from build123d import *

# Parameters (mm, degrees)
EXTRUDE1_DEPTH          = 20.6375
EXTRUDE1_DEPTH_BACK     = 20.6375
SKETCH2_R               = 4.0005
SKETCH2_R_2             = 1.1938
CUT_EXTRUDE1_DEPTH      = 20.6375
CUT_EXTRUDE1_DEPTH_BACK = 20.6375
SKETCH3_R               = 1.1938
CUT_EXTRUDE2_DEPTH      = 23.62886
CUT_EXTRUDE2_DEPTH_BACK = 23.62886
FILLET1_R               = 1.5875


with BuildPart() as part:
    # Sketch1 → Extrude1 (new body, two sides)
    with BuildSketch(Plane(origin=(0, 0, 0), x_dir=(0, 0, -1), z_dir=(1, 0, 0))) as extrude1_sk:
        with BuildLine():
            Line((-20.85086, 0), (20.85086, 0))
            ThreePointArc((20.85086, 0), (22.108095857, 0.520764143), (22.62886, 1.778))
            Line((22.62886, 1.778), (22.62886, 23.8252))
            Line((22.62886, 23.8252), (21.10486, 23.8252))
            Line((21.10486, 23.8252), (21.10486, 1.778))
            ThreePointArc((21.10486, 1.778), (21.030465122, 1.598394878), (20.85086, 1.524))
            Line((20.85086, 1.524), (-20.85086, 1.524))
            ThreePointArc((-20.85086, 1.524), (-21.030465122, 1.598394878), (-21.10486, 1.778))
            Line((-21.10486, 1.778), (-21.10486, 23.8252))
            Line((-21.10486, 23.8252), (-22.62886, 23.8252))
            Line((-22.62886, 23.8252), (-22.62886, 1.778))
            ThreePointArc((-22.62886, 1.778), (-22.108095857, 0.520764143), (-20.85086, 0))
        make_face()
    extrude(amount=EXTRUDE1_DEPTH)
    extrude(extrude1_sk.sketch, amount=-EXTRUDE1_DEPTH_BACK)

    # Sketch2 → Cut-Extrude1 (cut, two sides)
    with BuildSketch(Plane(origin=(0, 0, 0), x_dir=(1, 0, 0), z_dir=(0, 1, 0))) as cut_extrude1_sk:
        with Locations(Location((-8.3312, 0, 0), (0, 0, 270))):  # turned: the seam where the file's is
            Circle(SKETCH2_R)
        with Locations(Location((8.3312, 0, 0), (0, 0, 270))):  # turned: the seam where the file's is
            Circle(SKETCH2_R)
        with Locations(Location((16.6624, 0, 0), (0, 0, 270))):  # turned: the seam where the file's is
            Circle(SKETCH2_R_2)
        with Locations(Location((-16.6624, 0, 0), (0, 0, 270))):  # turned: the seam where the file's is
            Circle(SKETCH2_R_2)
        with Locations(Location((-8.3312, 8.3312, 0), (0, 0, 270))):  # turned: the seam where the file's is
            Circle(SKETCH2_R_2)
        with Locations(Location((8.3312, 8.3312, 0), (0, 0, 270))):  # turned: the seam where the file's is
            Circle(SKETCH2_R_2)
        with Locations(Location((-8.3312, -8.3312, 0), (0, 0, 270))):  # turned: the seam where the file's is
            Circle(SKETCH2_R_2)
        with Locations(Location((8.3312, -8.3312, 0), (0, 0, 270))):  # turned: the seam where the file's is
            Circle(SKETCH2_R_2)
        with Locations(Location((0, 0, 0), (0, 0, 270))):  # turned: the seam where the file's is
            Circle(SKETCH2_R_2)
    extrude(amount=CUT_EXTRUDE1_DEPTH, mode=Mode.SUBTRACT)
    extrude(cut_extrude1_sk.sketch, amount=-CUT_EXTRUDE1_DEPTH_BACK, mode=Mode.SUBTRACT)

    # Sketch3 → Cut-Extrude2 (cut, two sides)
    with BuildSketch(Plane.XY) as cut_extrude2_sk:
        with Locations((-17.8689, 13.8938)):
            Circle(SKETCH3_R)
        with Locations((-9.9187, 13.8938)):
            Circle(SKETCH3_R)
        with Locations((9.9187, 13.8938)):
            Circle(SKETCH3_R)
        with Locations((17.8689, 13.8938)):
            Circle(SKETCH3_R)
    extrude(amount=CUT_EXTRUDE2_DEPTH, mode=Mode.SUBTRACT)
    extrude(cut_extrude2_sk.sketch, amount=-CUT_EXTRUDE2_DEPTH_BACK, mode=Mode.SUBTRACT)

    # Fillet1
    fillet1_edges = [part.edges().sort_by_distance(p)[0] for p in [
        (20.6375, 23.8252, -21.86686),
        (-20.6375, 23.8252, 21.86686),
        (-20.6375, 23.8252, -21.86686),
        (20.6375, 23.8252, 21.86686),
    ]]
    fillet(fillet1_edges, radius=FILLET1_R)


solid = part.part
Design review of the part built by this model. Coordinates are the model's own, in mm. A direction names the side the tool comes from. Coordinates: 2 decimals unless noted, no trailing zeros. Write each loop counter-clockwise with the first axis right and the second up, starting at its lowest first coordinate (ties: lowest second). Pieces come first, ordered by that corner, then holes. Notation, with made-up numbers: (70.5, 66) -> (129.5, 66) arc R25 ccw to (129.5, 98) -> close; hole circle Ø4 at (-28.75, -10.5). An arc over 180 degrees is marked (long way). Write each question's results on one line, items separated by ' | '. Start each with the question number.
(1) For line 1 along Z through (x, y) = (18.5, 17.5); line 2 along Y through (x, z) = (15.5, 1); line 3 along Y through (x, z) = (8, 21.5), list the stretches that pass through material, from the lowest coordinate up. Write a range as from..to.
(2) Tool access review of faces 1 (the face through (12.3, 0.8, -0.5)), 2 (the face through (0, 13, 21.105)): name each direction out of +Z, -Z, +X, -X, +Y, -Y from which nothing blocks a thin tool from reaching the whole face with its end or side.
(3) Take a section at A-A on y = 3. Write out the cut boundary in (x, z).
(4) Take a section at B-B on x = 0. Write out the cut boundary in (y, z).
(5) Clearance check with flat-ended pins moving along their axes: P1, Ø1.9, axis at x = -8.33, z = 8.33, coming from the +Y side; P2, Ø12, axis at x = -15.5, z = -10, coming from the +Y side; P3, Ø2.5, axis at x = 9.92, y = 13.89, coming from the -Z side. State where each tip first meets the part, or that it passes through.
(6) The part is to be moulded in two halves that separate along Z. For faces 3 (the face through (20.18, 23.35, -21.86)), 4 (the face through (8.69, 0.751, -7.193)), 5 (the face through (0, 13, 22.629)), say which applies: pulls with the +Z half, pulls with the -Z half, needs draft (parallel to the pull), parting line crosses it, or undercut.
(7) Take a section at C-C on z = 0. Write out the cut boundary in (x, y).
(8) Take a section at D-D on z = -13. Write out the cut boundary in (x, y).
Results found:
1) line 1: z = -22.63..-21.1, 21.1..22.63 | line 2: y = 0..1.52 | line 3: y = 0.12..23.83
2) face 1: +Y, -Y | face 2: +X, -X, +Y
3) outline: (-20.64, -22.63) -> (20.64, -22.63) -> (20.64, -21.1) -> (-20.64, -21.1) -> close; (-20.64, 21.1) -> (20.64, 21.1) -> (20.64, 22.63) -> (-20.64, 22.63) -> close
4) outline: (0, -20.85) arc R1.78 ccw to (1.78, -22.63) -> (23.83, -22.63) -> (23.83, -21.1) -> (1.78, -21.1) arc R0.25 cw to (1.52, -20.85) -> (1.52, -1.19) -> (0, -1.19) -> close; (0, 1.19) -> (1.52, 1.19) -> (1.52, 20.85) arc R0.25 cw to (1.78, 21.1) -> (23.83, 21.1) -> (23.83, 22.63) -> (1.78, 22.63) arc R1.78 ccw to (0, 20.85) -> close
5) P1: passes through | P2: stops at y = 1.52 | P3: stops at z = -22.63
6) face 3: needs draft | face 4: undercut | face 5: pulls with the +Z half
7) outline: (-20.64, 0) -> (-17.86, 0) -> (-17.86, 1.52) -> (-20.64, 1.52) -> close; (-15.47, 0) -> (-12.33, 0) -> (-12.33, 1.52) -> (-15.47, 1.52) -> close; (-4.33, 0) -> (-1.19, 0) -> (-1.19, 1.52) -> (-4.33, 1.52) -> close; (1.19, 0) -> (4.33, 0) -> (4.33, 1.52) -> (1.19, 1.52) -> close; (12.33, 0) -> (15.47, 0) -> (15.47, 1.52) -> (12.33, 1.52) -> close; (17.86, 0) -> (20.64, 0) -> (20.64, 1.52) -> (17.86, 1.52) -> close
8) outline: (-20.64, 0) -> (20.64, 0) -> (20.64, 1.52) -> (-20.64, 1.52) -> close
